from build123d import *

# Parameters (mm, degrees)
SKETCH1_R               = 8.5
SKETCH1_R_2             = 7
BOSS_EXTRUDE1_DEPTH     = 6
SKETCH2_R               = 8.5
BOSS_EXTRUDE2_DEPTH     = 0.75
CUT_EXTRUDE1_DEPTH      = 14.786315679
CUT_EXTRUDE1_DEPTH_BACK = 14.786315679
SKETCH3_R               = 0.625
FILLET1_R               = 0.5


with BuildPart() as part:
    # Sketch1 → Boss-Extrude1 (new body)
    with BuildSketch(Plane(origin=(0, 0, 0), x_dir=(1, 0, 0), z_dir=(0, 1, 0))):
        with Locations(Location((0, 0, 0), (0, 0, 270))):
            Circle(SKETCH1_R)
        with Locations(Location((0, 0, 0), (0, 0, 270))):
            Circle(SKETCH1_R_2, mode=Mode.SUBTRACT)
    extrude(amount=BOSS_EXTRUDE1_DEPTH)

    # Sketch2 → Boss-Extrude2 (add)
    with BuildSketch(Plane(origin=(0, 6, 0), x_dir=(1, 0, 0), z_dir=(0, 1, 0))):
        with Locations(Location((0, 0, 0), (0, 0, 270))):
            Circle(SKETCH2_R)
    extrude(amount=BOSS_EXTRUDE2_DEPTH)

    # Sketch3 → Cut-Extrude1 (cut, two sides: drawn at the far end of the back side and taken through both)
    with BuildSketch(Plane(origin=(0, 6.75, 0), x_dir=(1, 0, 0), z_dir=(0, 1, 0)).offset(-CUT_EXTRUDE1_DEPTH_BACK)):
        with Locations(Location((0, 0, 0), (0, 0, 270))):
            Circle(SKETCH3_R)
    extrude(amount=CUT_EXTRUDE1_DEPTH + CUT_EXTRUDE1_DEPTH_BACK, mode=Mode.SUBTRACT)

    # Fillet1
    fillet1_edges = [part.edges().sort_by_distance(p)[0] for p in [
        (0, 0, -7),
    ]]
    fillet(fillet1_edges, radius=FILLET1_R)


solid = part.part
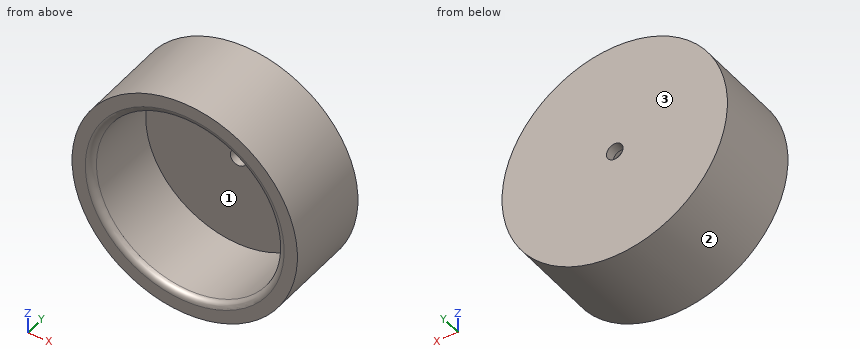
Design review of the part built by this model. Coordinates are the model's own, in mm. Face numbers are marked on the shaded views. Coordinates: 2 decimals unless noted, no trailing zeros. Loops run counter-clockwise (first coordinate to the right, second up) from the corner with the lowest first, then second, coordinate; pieces in that order, holes last. Notation, with made-up numbers: M -26.5,24.25 L -13.5,24.25 A30 cw -13.5,47.25 Z; hole C 35.5,22.5 d1. An arc over 180 degrees is marked long. Answer as CSV lines item,"result".
Item 1: For probe 1 along X at (y, z) = (6.3, 0) (3 decimals); probe 2 along Z at (x, y) = (0.25, 1.5), list the stretches that pass through material, from the lowest coordinate up.
Answer list:
probe 1,"-8.5 to -0.625, 0.625 to 8.5"
probe 2,"-8.5 to -7, 7 to 8.5"
Item 2: For P1, Ø4, axis at x = 3.5, z = 1.5, coming from the -Y side; P2, Ø1, axis at x = -6, y = 4.5, coming from the +Z side; P3, Ø2, axis at y = 1, z = -1.5, coming from the -X side, all flat-tipped, find the tip position at first contact; note any pin that passes through.
Answer list:
P1,"y = 6"
P2,"z = 6.48"
P3,"x = -8.49"
Item 3: Add section C-C on y = 5.25. State the section outline as (x, z) points, plus the area to 3 significant figures.
Answer list:
outline,"C 0,0 d17; hole C 0,0 d14"
area,"73.0 mm²"
Item 4: Add section A-A on x = 0. State the section outline as (y, z) points (3 decimals).
Answer list:
outline,"M 0,-8.5 L 6.75,-8.5 L 6.75,-0.625 L 6,-0.625 L 6,-7 L 0.5,-7 A0.5 ccw 0,-7.5 Z; M 0,7.5 A0.5 ccw 0.5,7 L 6,7 L 6,0.625 L 6.75,0.625 L 6.75,8.5 L 0,8.5 Z"
Item 5: Add section B-B on z = 0. State the section outline as (x, y) points (3 decimals).
Answer list:
outline,"M -8.5,0 L -7.5,0 A0.5 ccw -7,0.5 L -7,6 L -0.625,6 L -0.625,6.75 L -8.5,6.75 Z; M 0.625,6 L 7,6 L 7,0.5 A0.5 ccw 7.5,0 L 8.5,0 L 8.5,6.75 L 0.625,6.75 Z"
Item 6: The part is to be moulded in two halves that separate along X. For the marked faces 1, 2 and 3, say which applies: pulls with the +X half, pulls with the -X half, needs draft (parallel to the pull), parting line crosses it, or undercut.
Answer list:
face 1,"undercut"
face 2,"parting line crosses it"
face 3,"needs draft"
